from build123d import *

# Parameters (mm, degrees)
F0_W     = 10
F0_H     = 40
F1_DEPTH = 3
F2_DEPTH = 10
F4_DEPTH = 56
F5_DEPTH = 10
F6_START = -7
F0_R     = 1.75
F6_DEPTH = 3
F7_R     = 3.2


with BuildPart() as f1:
    # F0 (on Top) → F1 (new body)
    with BuildSketch(Plane.XY):
        with Locations((0, 14.3)):
            Rectangle(F0_W, F0_H)
        Polygon((-28, 14.3), (-28, -5.7), (-24.5, -5.7), (-24.5, -4.2), (-19.5, -4.2), (-19.5, -5.7), (-13.5, -5.7), (-13.5, -4.2), (-8.5, -4.2), (-8.5, -5.7), (-5, -5.7), (-5, 34.3), (-8.5, 34.3), (-8.5, 32.8), (-13.5, 32.8), (-13.5, 34.3), (-19.5, 34.3), (-19.5, 32.8), (-24.5, 32.8), (-24.5, 34.3), (-28, 34.3), align=None)
        Polygon((24.5, -5.7), (28, -5.7), (28, 34.3), (24.5, 34.3), (24.5, 32.8), (19.5, 32.8), (19.5, 34.3), (13.5, 34.3), (13.5, 32.8), (8.5, 32.8), (8.5, 34.3), (5, 34.3), (5, -5.7), (8.5, -5.7), (8.5, -4.2), (13.5, -4.2), (13.5, -5.7), (19.5, -5.7), (19.5, -4.2), (24.5, -4.2), align=None)
    extrude(amount=F1_DEPTH)

    # F0 (on Top) → F2 (join)
    with BuildSketch(Plane.XY):
        Polygon((-28, 14.3), (-28, -5.7), (-24.5, -5.7), (-24.5, -4.2), (-19.5, -4.2), (-19.5, -5.7), (-13.5, -5.7), (-13.5, -4.2), (-8.5, -4.2), (-8.5, -5.7), (-5, -5.7), (-5, 34.3), (-8.5, 34.3), (-8.5, 32.8), (-13.5, 32.8), (-13.5, 34.3), (-19.5, 34.3), (-19.5, 32.8), (-24.5, 32.8), (-24.5, 34.3), (-28, 34.3), align=None)
        Polygon((24.5, -5.7), (28, -5.7), (28, 34.3), (24.5, 34.3), (24.5, 32.8), (19.5, 32.8), (19.5, 34.3), (13.5, 34.3), (13.5, 32.8), (8.5, 32.8), (8.5, 34.3), (5, 34.3), (5, -5.7), (8.5, -5.7), (8.5, -4.2), (13.5, -4.2), (13.5, -5.7), (19.5, -5.7), (19.5, -4.2), (24.5, -4.2), align=None)
    extrude(amount=-F2_DEPTH)

    # F3 (on face) → F4 (cut, through all)
    with BuildSketch(Plane.YZ.offset(28)):
        with BuildLine():
            Line((-1.5113883008, -10), (30.1113883008, -10))
            ThreePointArc((30.1113883008, -10), (14.3, 0), (-1.5113883008, -10))
        make_face()
    extrude(amount=-F4_DEPTH, mode=Mode.SUBTRACT)

    # F0 (on Top) → F5 (join, through all)
    with BuildSketch(Plane.XY):
        with Locations((0, 14.3)):
            Rectangle(F0_W, F0_H)
    extrude(amount=-F5_DEPTH)

    # F0 (on Top) → F6 (join)
    with BuildSketch(Plane.XY.offset(F6_START)):
        Polygon((-28, 37.5), (-28, 34.3), (-24.5, 34.3), (-24.5, 35.8), (-19.5, 35.8), (-19.5, 34.3), (-13.5, 34.3), (-13.5, 35.8), (-8.5, 35.8), (-8.5, 34.3), (-5, 34.3), (5, 34.3), (8.5, 34.3), (8.5, 35.8), (13.5, 35.8), (13.5, 34.3), (19.5, 34.3), (19.5, 35.8), (24.5, 35.8), (24.5, 34.3), (28, 34.3), (28, 37.5), align=None)
        Polygon((-28, -5.7), (-28, -8.9), (-6, -8.9), (-6, -8), (6, -8), (6, -8.9), (28, -8.9), (28, -5.7), (24.5, -5.7), (24.5, -7.2), (19.5, -7.2), (19.5, -5.7), (13.5, -5.7), (13.5, -7.2), (8.5, -7.2), (8.5, -5.7), (5, -5.7), (-5, -5.7), (-8.5, -5.7), (-8.5, -7.2), (-13.5, -7.2), (-13.5, -5.7), (-19.5, -5.7), (-19.5, -7.2), (-24.5, -7.2), (-24.5, -5.7), align=None)
        Polygon((-50, -37.5), (-28, -37.5), (0, -37.5), (28, -37.5), (50, -37.5), (50, -8.9), (28, -8.9), (6, -8.9), (6, -16), (-6, -16), (-6, -8.9), (-28, -8.9), (-50, -8.9), align=None)
        with Locations((-10, -32.5)):
            Circle(F0_R, mode=Mode.SUBTRACT)
        with Locations((-46.8, -12.1)):
            Circle(F0_R, mode=Mode.SUBTRACT)
        with Locations((10, -32.5)):
            Circle(F0_R, mode=Mode.SUBTRACT)
        with Locations((29.375, -33.055)):
            Circle(F0_R, mode=Mode.SUBTRACT)
    extrude(amount=-F6_DEPTH)

    # F7
    f7_edges = [f1.edges().sort_by_distance(p)[0] for p in [
        (28, 37.5, -8.5),
        (-28, 37.5, -8.5),
        (50, -8.9, -8.5),
        (50, -37.5, -8.5),
        (-50, -37.5, -8.5),
        (-50, -8.9, -8.5),
    ]]
    fillet(f7_edges, radius=F7_R)


solid = f1.part
Work out the finished part from the listing and answer in its coordinate system (mm). A direction names the side the tool comes from. Coordinates: 2 decimals unless noted, no trailing zeros. Loops run counter-clockwise (first coordinate to the right, second up) from the corner with the lowest first, then second, coordinate; pieces in that order, holes last. Notation, with made-up numbers: (2, -5) -> (42, -5) arc R19 cw to (42, 4) -> close; hole circle Ø8 at (62.5, -28.75). An arc over 180 degrees is marked (long way). Write each question's results on one line, items separated by ' | '. Start each with the question number.
1) Consider line 1 along X through (y, z) = (-15, -8.5); line 2 along Y through (x, z) = (-10, -7.95); line 3 along Y through (x, z) = (-46.8, -8.1). Determine where each line is inside the solid, lowest interval first.
2) Find section C-C on x = 35. Determine the outline of the cut face in (y, z), then the cut area to 3 significant figures.
3) Find section D-D on z = -8.5. Count the separate pieces of the cut face and the enclosed holes in it, then the cut area to 3 significant figures.
4) Find section B-B on y = 9.5. Determine the outline of the cut face in (x, z).
5) The mould has two halves that part along Y. Classify faces 1 (the cylindrical face through (49.087, -36.538, -8.521)), 2 (the flat face through (11, 35.8, -8)), 3 (the flat face through (-28, 13, 1)), 4 (the cylindrical face through (-27.087, 36.538, -8.521)): pulls with the +Y half, pulls with the -Y half, needs draft (parallel to the pull), parting line crosses it, or undercut.
6) Flat-ended cylindrical pins translate along their axes: P1, Ø3.5, axis at y = 34.5, z = -1.5, coming from the -X side; P2, Ø1, axis at x = -26.5, z = -2.5, coming from the -Y side; P3, Ø3, axis at x = -2.5, z = -1.5, coming from the +Y side. Find the tip coordinate at first contact, or state that the pin passes through.
7) Find section A-A on x = -10. Determine the outline of the cut face in (y, z).
8) For faces 5 (the flat face through (38, -8.9, -8)), 6 (the flat face through (11, -7.2, -8)), 7 (the flat face through (-26, 34.3, -2)), determine the directions among +Z, -Z, +X, -X, +Y, -Y from which every point of the face is accessible in a straight line to the end or side of a thin tool.
Response values:
1) line 1: x = -50 to -6, 6 to 50 | line 2: y = -37.5 to -34.25, -30.75 to -7.2, -4.2 to -0.36, 28.96 to 32.8, 35.8 to 37.5 | line 3: y = -37.5 to -13.85, -10.35 to -8.9
2) outline: (-37.5, -10) -> (-8.9, -10) -> (-8.9, -7) -> (-37.5, -7) -> close | area: 85.8 mm^2
3) separate pieces: 1 | enclosed holes: 13 | area: 3,810 mm^2
4) outline: (-28, -0.67) -> (-5, -0.67) -> (-5, -10) -> (5, -10) -> (5, -0.67) -> (28, -0.67) -> (28, 3) -> (-28, 3) -> close
5) face 1: pulls with the -Y half | face 2: undercut | face 3: needs draft | face 4: pulls with the +Y half
6) P1: stops at x = -28 | P2: stops at y = -5.7 | P3: stops at y = 34.3
7) outline: (-37.5, -10) -> (-34.25, -10) -> (-34.25, -7) -> (-37.5, -7) -> close; (-30.75, -10) -> (-7.2, -10) -> (-7.2, -7) -> (-30.75, -7) -> close; (-4.2, -10) -> (-1.51, -10) arc R17.5 cw to (30.11, -10) -> (32.8, -10) -> (32.8, 3) -> (-4.2, 3) -> close; (35.8, -10) -> (37.5, -10) -> (37.5, -7) -> (35.8, -7) -> close
8) face 5: +Z, -Z, +X, +Y | face 6: +Z, -Z | face 7: +Z, +X, -X, +Y
